```python
from build123d import *

# Parameters (mm, degrees)
SKETCH1_W           = 28
SKETCH1_H           = 35
SKETCH1_R           = 1.5
BOSS_EXTRUDE1_DEPTH = 2
SKETCH2_W           = 9.803487011
SKETCH2_H           = 7.411177961
BOSS_EXTRUDE2_DEPTH = 6
SKETCH2_3_W         = 5
SKETCH2_3_H         = 15
BOSS_EXTRUDE3_DEPTH = 3
SKETCH2_4_R         = 1.188771684
SKETCH2_4_R_2       = 1.358321726
BOSS_EXTRUDE4_DEPTH = 4
SKETCH2_5_W         = 3.990758571
SKETCH2_5_H         = 2.149147788
SKETCH2_5_W_2       = 2.114664683
SKETCH2_5_H_2       = 1.232229244
SKETCH2_5_W_3       = 3.092189454
SKETCH2_5_H_3       = 1.517885082
SKETCH2_5_H_4       = 1.341337727
SKETCH2_5_W_4       = 1.043883653
SKETCH2_5_H_5       = 2.549502456
SKETCH2_5_W_5       = 0.955721455
SKETCH2_5_H_6       = 1.716190389
BOSS_EXTRUDE5_DEPTH = 1
FILLET1_R           = 1
SKETCH3_R           = 2.5
CUT_EXTRUDE1_DEPTH  = 6


with BuildPart() as part:
    # Sketch1 → Boss-Extrude1 (new body)
    with BuildSketch(Plane(origin=(0, 0, 0), x_dir=(1, 0, 0), z_dir=(0, 1, 0))):
        with Locations((14, 17.5)):
            Rectangle(SKETCH1_W, SKETCH1_H)
        with Locations((2.5, 2)):
            Circle(SKETCH1_R, mode=Mode.SUBTRACT)
        with Locations((2.5, 33)):
            Circle(SKETCH1_R, mode=Mode.SUBTRACT)
    extrude(amount=BOSS_EXTRUDE1_DEPTH)

    # Sketch2 → Boss-Extrude2 (add)
    with BuildSketch(Plane(origin=(0, 2, 0), x_dir=(1, 0, 0), z_dir=(0, 1, 0))):
        with Locations((23.098256494, 9.79441102)):
            Rectangle(SKETCH2_W, SKETCH2_H)
    extrude(amount=-BOSS_EXTRUDE2_DEPTH)

    # Sketch2<3> → Boss-Extrude3 (add)
    with BuildSketch(Plane(origin=(0, 2, 0), x_dir=(1, 0, 0), z_dir=(0, 1, 0))):
        with Locations((9.343972274, 15.538611718)):
            Rectangle(SKETCH2_3_W, SKETCH2_3_H)
    extrude(amount=BOSS_EXTRUDE3_DEPTH)

    # Sketch2<4> → Boss-Extrude4 (add)
    with BuildSketch(Plane(origin=(0, 2, 0), x_dir=(1, 0, 0), z_dir=(0, 1, 0))):
        with Locations((10.43268107, 3.363069922)):
            Circle(SKETCH2_4_R)
        with Locations((24.262223339, 20.185094641)):
            Circle(SKETCH2_4_R_2)
    extrude(amount=BOSS_EXTRUDE4_DEPTH)

    # Sketch2<5> → Boss-Extrude5 (add)
    with BuildSketch(Plane(origin=(0, 2, 0), x_dir=(1, 0, 0), z_dir=(0, 1, 0))):
        with Locations((9.848592989, 30.151261091)):
            Rectangle(SKETCH2_5_W, SKETCH2_5_H)
        with Locations((18.212826519, 31.841949607)):
            Rectangle(SKETCH2_5_W_2, SKETCH2_5_H_2)
        with Locations((20.816253587, 26.392524838)):
            Rectangle(SKETCH2_5_W_3, SKETCH2_5_H_3)
        with Locations((18.212826519, 20.855763505)):
            Rectangle(SKETCH2_5_W_2, SKETCH2_5_H_4)
        with Locations((15.671715961, 8.251316283)):
            Rectangle(SKETCH2_5_W_4, SKETCH2_5_H_5)
        with Locations((2.447985743, 25.534429644)):
            Rectangle(SKETCH2_5_W_5, SKETCH2_5_H_6)
    extrude(amount=BOSS_EXTRUDE5_DEPTH)

    # Fillet1
    fillet1_edges = [part.edges().sort_by_distance(p)[0] for p in [
        (0, 1, -35),
        (0, 1, 0),
    ]]
    fillet(fillet1_edges, radius=FILLET1_R)

    # Sketch3 → Cut-Extrude1 (cut)
    with BuildSketch(Plane(origin=(28, 0, 0), x_dir=(0, 0, -1), z_dir=(1, 0, 0))):
        with Locations((9.8, -1)):
            Circle(SKETCH3_R)
    extrude(amount=-CUT_EXTRUDE1_DEPTH, mode=Mode.SUBTRACT)


solid = part.part
```
Here's how the part is built. I have some questions about the finished solid (model axes, mm). A direction names the side the tool comes from. Give positions to 0.01 mm unless a question says otherwise; leave off trailing zeros. Loops run counter-clockwise (first coordinate to the right, second up) from the corner with the lowest first, then second, coordinate; pieces in that order, holes last. Notation, with made-up numbers: (57.25, -2) -> (76.25, -2) arc R24 cw to (76.25, 19) -> close; hole circle Ø10 at (72, -33). An arc over 180 degrees is marked (long way). Use one line per item in the form item = value. Start each with the question number.
1) Please list where these lines run through material, in increasing order: line 1 along Z through (x, y) = (2.5, 0.75); line 2 along Y through (x, z) = (25.3, -9.8); line 3 along X through (y, z) = (0.8, -2).
2) Imagine slicing it at C-C (y = -1). Please give me the cut outline in (x, z).
3) For P1, Ø0.8, axis at y = 2.5, z = -7.5, coming from the +X side; P2, Ø3, axis at x = 15, z = -20, coming from the -Y side; P3, Ø0.5, axis at x = 9.5, y = 2.5, coming from the -Z side, each with a flat end and sliding along its axis, tell me the tip position at first contact or that it passes through.
4) Imagine slicing it at D-D (z = -17.5). Please give me the cut outline in (x, y).
5) Imagine slicing it at A-A (x = 2.5). Please give me the cut outline in (y, z), then the cut area to 3 significant figures.
6) Imagine slicing it at B-B (z = -33). Please give me the cut outline in (x, y), then the cut area to 3 significant figures.
7) Thinking about a two-plate mould opening in Z: for faces 4 (the face through (19.27, 2.5, -20.8)), 5 (the face through (19.27, 2.5, -26.4)), 6 (the face through (20.8, 2.5, -25.634)), which applies, +Z half, -Z half, draft (parallel to the pull), parting line (faces both ways), or undercut?
8) Which directions (+Z, -Z, +X, -X, +Y, -Y) give clear straight access to the entire face, cutting with the end or side of a thin tool? Please do faces 1 (the face through (23.97, 3.97, -18.86)), 2 (the face through (17.155, 2.5, -31.8)), 3 (the face through (18.197, -2, -10)).
Check values:
q1.line_1 = -35 to -34.5, -31.5 to -3.5, -0.5 to 0
q1.line_2 = -4 to -3.5, 1.5 to 2
q1.line_3 = 0 to 1, 4 to 28
q2.outline = (18.2, -13.5) -> (28, -13.5) -> (28, -12.3) -> (22, -12.3) -> (22, -7.3) -> (28, -7.3) -> (28, -6.09) -> (18.2, -6.09) -> close
q3.P1 = 16.19
q3.P2 = 0
q3.P3 = -31.23
q4.outline = (0, 0) -> (28, 0) -> (28, 2) -> (11.84, 2) -> (11.84, 5) -> (6.84, 5) -> (6.84, 2) -> (0, 2) -> close
q5.outline = (0, -35) -> (2, -35) -> (2, -34.5) -> (0, -34.5) -> close; (0, -31.5) -> (2, -31.5) -> (2, -26.39) -> (3, -26.39) -> (3, -24.68) -> (2, -24.68) -> (2, -3.5) -> (0, -3.5) -> close; (0, -0.5) -> (2, -0.5) -> (2, 0) -> (0, 0) -> close
q5.area = 59.7 mm^2
q6.outline = (0, 0) -> (1, 0) -> (1, 2) -> (0, 2) -> close; (4, 0) -> (28, 0) -> (28, 2) -> (4, 2) -> close
q6.area = 50.0 mm^2
q7.face_4 = draft
q7.face_5 = undercut
q7.face_6 = +Z half
q8.face_1 = +Y
q8.face_2 = +Z, -Z, -X, +Y
q8.face_3 = +Z, -Z, -X, -Y
